Autodesk Fusion 360 part; units mm, degrees
sketch "Sketch1" plane through (0, 0, 0) normal (0, 0, 1) x (1, 0, 0)
  circle A0 centre (0, 0) radius 5.15
  circle A1 centre (0, 0) radius 7
  circle A2 centre (9, 0) radius 2.5
  circle A3 centre (-9, 0) radius 2.5
  circle A4 centre (-9, 0) radius 1.75
  circle A5 centre (9, 0) radius 1.75
  line L0 (-10.25, 2.1651) -> (-3.5, 6.0622)
  line L1 (-9, 0) -> (9, 0)
  line L2 (-10.25, -2.1651) -> (-3.5, -6.0622)
  line L3 (0, 12) -> (0, 15)
  line L4 (10.25, 2.1651) -> (3.5, 6.0622)
  line L5 (10.25, -2.1651) -> (3.5, -6.0622)
  dimension "d1" = 10.3
  dimension "d2" = 14
  dimension "d3" = 5
  dimension "d4" = 5
  dimension "d5" = 9
  dimension "d6" = 9
  dimension "d7" = 3.5
  dimension "d8" = 3.5
extrude "Extrude1" add sketch "Sketch1" along normal blind 5 contours A0 A1 A2 A3 L1 | A0 A1 A2 A3 L1 | A1 A2 L1 | A1 A2 L1 | A1 A3 L1 | A1 A3 L1 | A1 A2 | A1 A2 L4 | A1 A2 L5 | A1 A3 L0 | A1 A3 | A1 A3 L2
sketch "Sketch2" plane through (0, 0, 5) normal (0, 0, 1) x (-1, 0, 0)
  circle A0 centre (-9, 0) radius 1.75
  circle A1 centre (0, 0) radius 5.15
  circle A2 centre (9, 0) radius 1.75
  line L0 (-10.25, -2.1651) -> (-3.5, -6.0622)
  arc A3 (-3.5, -6.0622) -> (3.5, -6.0622) centre (0, 0) ccw
  line L1 (3.5, -6.0622) -> (10.25, -2.1651)
  arc A4 (10.25, -2.1651) -> (10.25, 2.1651) centre (9, 0) ccw
  line L2 (10.25, 2.1651) -> (3.5, 6.0622)
  arc A5 (3.5, 6.0622) -> (-3.5, 6.0622) centre (0, 0) ccw
  line L3 (-3.5, 6.0622) -> (-10.25, 2.1651)
  arc A6 (-10.25, 2.1651) -> (-10.25, -2.1651) centre (-9, 0) ccw
  circle A7 centre (0, 0) radius 3.15
  dimension "d11" = -2
extrude "Extrude2" add sketch "Sketch2" against normal blind 1 contours A1
Input: part model. Units: mm. Frame: model coordinates. A direction names the side the tool comes from. Coordinates: 2 decimals unless noted, no trailing zeros. Order: outer loops, then holes, each group sorted by start corner. A loop starts at its lowest first (then second) coordinate and runs counter-clockwise, first axis right, second up. Notation, with made-up numbers: M -7,51 L 22,51 A11 ccw 22,58 Z; hole C 81,58 d7. An arc over 180 degrees is marked long. Write item = value, one per line. Start each with the question number.
(1) Reachability of faces 4 (the flat face through (6.9, 4.1, 2.5)), 5 (the cylindrical face through (4.91, -1.55, 1.97)) from +Z, -Z, +X, -X, +Y, -Y: full face, straight path, thin tool, end or side. Return the list, or none.
(2) Section A-A on x = 0. Output: boundary loops of the cut face in (y, z).
(3) Line query: line 1 along Y through (x, z) = (0, 0.8); line 2 along X through (y, z) = (-0.5, 4.65); line 3 along X through (y, z) = (1.25, 2.55). Output: solid intervals per line, ascending. Write a range as [from, to].
(4) Section C-C on z = 4.25. Output: boundary loops of the cut face in (x, y), and give its area (3 significant figures).
(5) Section D-D on y = 2.75. Output: boundary loops of the cut face in (x, z).
(6) First-contact query: P1, Ø3, axis at y = -3.5, z = 3, coming from the +X side; P2, Ø8, axis at x = -1, y = -0.5, coming from the -Z side. Flat tips, straight axial feed; report the tip coordinate or a pass-through.
(7) Section B-B on y = 0. Output: boundary loops of the cut face in (x, z), and give its area (3 significant figures).
(8) Pull-direction query (X, two-part tool) for faces 1 (the cylindrical face through (2.5, 1.917, 4.507)), 2 (the cylindrical face through (0, -7, 2)), 3 (the flat face through (-6.9, -4.1, 2.5)); classes: released by +X, released by -X, zero draft, split by the parting line, or undercut.
Result set:
q1.face_4 = +Z, -Z, +X, +Y
q1.face_5 = -Z
q2.outline = M -7,0 L -5.15,0 L -5.15,4 L -3.15,4 L -3.15,5 L -7,5 Z; M 3.15,4 L 5.15,4 L 5.15,0 L 7,0 L 7,5 L 3.15,5 Z
q3.line_1 = [-7, -5.15], [5.15, 7]
q3.line_2 = [-11.45, -10.68], [-7.32, -3.11], [3.11, 7.32], [10.68, 11.45]
q3.line_3 = [-11.17, -10.22], [-7.78, -5], [5, 7.78], [10.22, 11.17]
q4.outline = M -10.25,-2.17 L -3.5,-6.06 A7 ccw 3.5,-6.06 L 10.25,-2.17 A2.5 ccw 10.25,2.17 L 3.5,6.06 A7 ccw -3.5,6.06 L -10.25,2.17 A2.5 ccw Z; hole C -9,0 d3.5; hole C 0,0 d6.3; hole C 9,0 d3.5
q4.area = 162 mm²
q5.outline = M -9.24,0 L -4.35,0 L -4.35,4 L -1.54,4 L -1.54,5 L -9.24,5 Z; M 1.54,4 L 4.35,4 L 4.35,0 L 9.24,0 L 9.24,5 L 1.54,5 Z
q6.P1 = 10.5
q6.P2 = 4
q7.outline = M -11.5,0 L -10.75,0 L -10.75,5 L -11.5,5 Z; M -7.25,0 L -5.15,0 L -5.15,4 L -3.15,4 L -3.15,5 L -7.25,5 Z; M 3.15,4 L 5.15,4 L 5.15,0 L 7.25,0 L 7.25,5 L 3.15,5 Z; M 10.75,0 L 11.5,0 L 11.5,5 L 10.75,5 Z
q7.area = 32.5 mm²
q8.face_1 = undercut
q8.face_2 = split by the parting line
q8.face_3 = released by -X
